Can you work these out from the model? Positions are in its coordinate system, mm. A direction names the side the tool comes from. Give positions to 0.01 mm unless a question says otherwise; leave off trailing zeros. Order: outer loops, then holes, each group sorted by start corner. A loop starts at its lowest first (then second) coordinate and runs counter-clockwise, first axis right, second up. Notation, with made-up numbers: (-30, -16.5) - (6, -16.5) arc R22 ccw to (6, 19.5) - close; hole circle Ø3 at (14, 77.5). An arc over 180 degrees is marked (long way). Answer as a JSON object with one key per item and string values.
```python
from build123d import *

# Parameters (mm, degrees)
SKETCH_W     = 10.2
SKETCH_H     = 8
SKETCH_W_2   = 9
SKETCH_H_2   = 6.8
PAD_DEPTH    = 8
SKETCH001_R  = 2.6
POCKET_DEPTH = 0.6
FILLET_R     = 0.2
FILLET001_R  = 0.2


with BuildPart() as part:
    # Sketch → Pad (new body)
    with BuildSketch(Plane.XZ):
        with Locations((5.1, 4)):
            Rectangle(SKETCH_W, SKETCH_H)
        with Locations((5.1, 4)):
            Rectangle(SKETCH_W_2, SKETCH_H_2, mode=Mode.SUBTRACT)
    extrude(amount=PAD_DEPTH)

    # Sketch001 (on Face1 of Pad) → Pocket (cut)
    with BuildSketch(Plane(origin=(0, 0, 0), x_dir=(1, 0, 0), z_dir=(0, 0, -1))):
        with Locations((5.1, 4)):
            Circle(SKETCH001_R)
    extrude(amount=-POCKET_DEPTH, mode=Mode.SUBTRACT)

    # Fillet
    fillet_edges = [part.edges().sort_by_distance(p)[0] for p in [
        (5.1, -8, 7.4),
        (0.6, -8, 4),
        (9.6, -8, 4),
        (5.1, -8, 0.6),
        (5.1, 0, 7.4),
        (9.6, 0, 4),
        (5.1, 0, 0.6),
        (0.6, 0, 4),
    ]]
    fillet(fillet_edges, radius=FILLET_R)

    # Fillet001
    fillet001_edges = [part.edges().sort_by_distance(p)[0] for p in [
        (0, -4, 8),
        (10.2, -4, 8),
        (0, -4, 0),
        (10.2, -4, 0),
    ]]
    fillet(fillet001_edges, radius=FILLET001_R)


solid = part.part
```
Q1. I'm going to push flat-ended pins straight in: pin 1 Ø3 at (x, y) = (5.1, -4) entering from -Z; pin 2 Ø1.5 at (x, z) = (8, 3.5) entering from -Y. Where does each tip first touch, or does it pass through?
Recorded:
{"pin 1": "stops at z = 7.4", "pin 2": "passes through"}
Q2. If we section it at C-C, the plane y = -4: Please give me the cut outline in (x, z).
Recorded:
{"outline": "(0, 0.2) arc R0.2 ccw to (0.2, 0) - (2.5, 0) - (2.5, 0.6) - (0.6, 0.6) - (0.6, 7.4) - (9.6, 7.4) - (9.6, 0.6) - (7.7, 0.6) - (7.7, 0) - (10, 0) arc R0.2 ccw to (10.2, 0.2) - (10.2, 7.8) arc R0.2 ccw to (10, 8) - (0.2, 8) arc R0.2 ccw to (0, 7.8) - close"}
Q3. Which directions (+Z, -Z, +X, -X, +Y, -Y) give clear straight access to the entire face, cutting with the end or side of a thin tool? Please do faces 1 (the face through (0.6, -4, 4)), 2 (the face through (5, -7, 0)).
Recorded:
{"face 1": "+Y, -Y", "face 2": "-Z, +X, -X, +Y, -Y"}
Q4. I need wall thicknesses on L1, parallel to Z at x = 8.5, y = -4.5; L2, parallel to X at y = -4, z = 6.5; L3, parallel to X at y = -4, z = 0.2. Which ranges of each line are inside material? Lowest first, please.
Recorded:
{"L1": "z = 0 to 0.6, 7.4 to 8", "L2": "x = 0 to 0.6, 9.6 to 10.2", "L3": "x = 0 to 2.5, 7.7 to 10.2"}
Q5. We'd pull the mould along X, two halves only. Please class faces 3 (the face through (10.2, -4, 4)), 4 (the face through (5, -4, 8)), 5 (the face through (7.58, -4.78, 0.3)), 6 (the face through (0, -4, 4)): released by +X, released by -X, zero draft, split by the parting line, or undercut.
Recorded:
{"face 3": "released by +X", "face 4": "zero draft", "face 5": "undercut", "face 6": "released by -X"}
Q6. If we section it at A-A, the plane z = 3.5: Please give me the cut outline in (x, y).
Recorded:
{"outline": "(0, -8) - (0.4, -8) arc R0.2 ccw to (0.6, -7.8) - (0.6, -0.2) arc R0.2 ccw to (0.4, 0) - (0, 0) - close; (9.6, -7.8) arc R0.2 ccw to (9.8, -8) - (10.2, -8) - (10.2, 0) - (9.8, 0) arc R0.2 ccw to (9.6, -0.2) - close"}
Q7. If we section it at B-B, the plane x = 5.1: Please give me the cut outline in (y, z).
Recorded:
{"outline": "(-8, 0) - (-6.6, 0) - (-6.6, 0.6) - (-7.8, 0.6) arc R0.2 ccw to (-8, 0.4) - close; (-8, 7.6) arc R0.2 ccw to (-7.8, 7.4) - (-0.2, 7.4) arc R0.2 ccw to (0, 7.6) - (0, 8) - (-8, 8) - close; (-1.4, 0) - (0, 0) - (0, 0.4) arc R0.2 ccw to (-0.2, 0.6) - (-1.4, 0.6) - close"}
Q8. If we section it at D-D, the plane x = 3.5: Please give me the cut outline in (y, z), then the cut area to 3 significant figures.
Recorded:
{"outline": "(-8, 0) - (-6.05, 0) - (-6.05, 0.6) - (-7.8, 0.6) arc R0.2 ccw to (-8, 0.4) - close; (-8, 7.6) arc R0.2 ccw to (-7.8, 7.4) - (-0.2, 7.4) arc R0.2 ccw to (0, 7.6) - (0, 8) - (-8, 8) - close; (-1.95, 0) - (0, 0) - (0, 0.4) arc R0.2 ccw to (-0.2, 0.6) - (-1.95, 0.6) - close", "area": "7.11 mm^2"}
